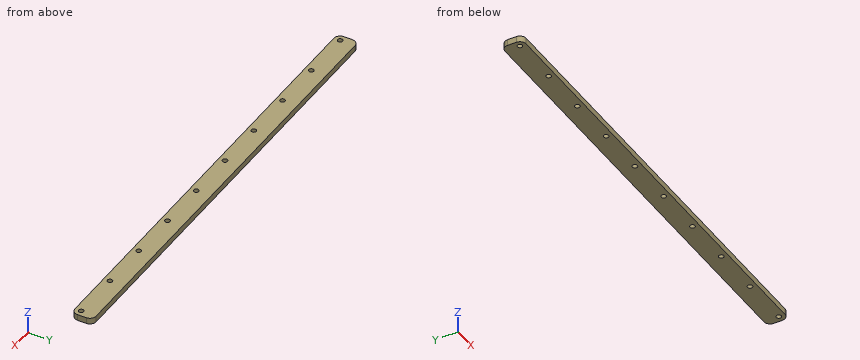
from build123d import *

# Parameters (mm, degrees)
ESQUISSE1_W        = 370
ESQUISSE1_H        = 17
ESQUISSE1_R        = 2
BOSS_EXTRU_1_DEPTH = 5
CONG_1_R           = 5


with BuildPart() as part:
    # Esquisse1 → Boss.-Extru.1 (new body)
    with BuildSketch(Plane.XY):
        with Locations((185, 8.5)):
            Rectangle(ESQUISSE1_W, ESQUISSE1_H)
        with Locations((5, 5)):
            Circle(ESQUISSE1_R, mode=Mode.SUBTRACT)
        with Locations((45, 5)):
            Circle(ESQUISSE1_R, mode=Mode.SUBTRACT)
        with Locations((85, 5)):
            Circle(ESQUISSE1_R, mode=Mode.SUBTRACT)
        with Locations((125, 5)):
            Circle(ESQUISSE1_R, mode=Mode.SUBTRACT)
        with Locations((165, 5)):
            Circle(ESQUISSE1_R, mode=Mode.SUBTRACT)
        with Locations((205, 5)):
            Circle(ESQUISSE1_R, mode=Mode.SUBTRACT)
        with Locations((245, 5)):
            Circle(ESQUISSE1_R, mode=Mode.SUBTRACT)
        with Locations((285, 5)):
            Circle(ESQUISSE1_R, mode=Mode.SUBTRACT)
        with Locations((325, 5)):
            Circle(ESQUISSE1_R, mode=Mode.SUBTRACT)
        with Locations((365, 5)):
            Circle(ESQUISSE1_R, mode=Mode.SUBTRACT)
    extrude(amount=BOSS_EXTRU_1_DEPTH)

    # Congé1
    cong_1_edges = [part.edges().sort_by_distance(p)[0] for p in [
        (0, 17, 2.5),
        (370, 17, 2.5),
        (370, 0, 2.5),
        (0, 0, 2.5),
    ]]
    fillet(cong_1_edges, radius=CONG_1_R)


solid = part.part
Geometry: final body of the model. Coordinates: model frame, mm. Give positions to 0.01 mm unless a question says otherwise; leave off trailing zeros. Return JSON: item names as keys, results as strings. Group by question number.
1) Section A-A on z = 2.9. State how many separate pieces and enclosed holes the cut face has, plus the area to 3 significant figures.
2) Line query: line 1 (Y direction, x = 85, z = 1.85); line 2 (X direction, y = 14, z = 4.15); line 3 (X direction, y = 0.75, z = 3.6). Output: solid intervals per line, ascending.
3) First-contact query: P1, Ø2.5, axis at x = 205, y = 5, coming from the -Z side; P2, Ø3, axis at y = 2.5, z = 2, coming from the -X side. Flat tips, straight axial feed; report the tip coordinate or a pass-through.
Filled in:
{
 "1": {"separate pieces": "1", "enclosed holes": "10", "area": "6,140 mm^2"},
 "2": {"line 1": "y = 0 to 3, 7 to 17", "line 2": "x = 0.42 to 369.58", "line 3": "x = 2.37 to 367.63"},
 "3": {"P1": "passes through", "P2": "stops at x = 0.1"}
}
